```python
from build123d import *

# Parameters (mm, degrees)
F0_R      = 12.7
F1_DEPTH  = 60.325
F2_R      = 3.302
F3_W      = 57.4852150798
F3_H      = 22.3266
F4_DEPTH  = 57.151
F3_W_2    = 22.8455264698
F3_H_2    = 41.275
F3_W_3    = 20.32
F3_W_4    = 13.4658747114
F5_DEPTH  = 34.798
F6_R      = 6.35
F7_DEPTH  = 22.353
F8_R      = 5.08
F9_R      = 7.874
F11_DEPTH = 19.05


with BuildPart() as f1:
    # F0 (on Front) → F1 (new body)
    with BuildSketch(Plane.XZ):
        with BuildLine():
            Line((117.2464, 0), (22.352, 0))
            ThreePointArc((22.352, 0), (-15.8052507731, 15.8052507731), (0, -22.352))
            Line((0, -22.352), (194.2084, -22.352))
            Line((194.2084, -22.352), (194.2084, 0))
            Line((194.2084, 0), (150.0886, 0))
            Line((150.0886, 0), (150.0886, 34.798))
            Line((150.0886, 34.798), (129.7686, 34.798))
            ThreePointArc((129.7686, 34.798), (126.786603396, 16.2190014787), (117.2464, 0))
        make_face()
        Circle(F0_R, mode=Mode.SUBTRACT)
    extrude(amount=F1_DEPTH)

    # F2
    f2_edges = [f1.edges().sort_by_distance(p)[0] for p in [
        (22.352, -30.1625, 0),
        (150.0886, -30.1625, 0),
    ]]
    fillet(f2_edges, radius=F2_R)

    # F3 (on face) → F4 (cut, through all)
    with BuildSketch(Plane.XY.offset(34.798)):
        with Locations((0, -30.1625)):
            Rectangle(F3_W, F3_H)
    extrude(amount=-F4_DEPTH, mode=Mode.SUBTRACT)

    # F3 (on face) → F5 (cut, through all)
    with BuildSketch(Plane.XY.offset(34.798)):
        with Locations((118.3458367651, -20.6375)):
            Rectangle(F3_W_2, F3_H_2)
        with Locations((139.9286, -20.6375)):
            Rectangle(F3_W_3, F3_H_2)
        with Locations((156.8215373557, -20.6375)):
            Rectangle(F3_W_4, F3_H_2)
    extrude(amount=-F5_DEPTH, mode=Mode.SUBTRACT)

    # F6 (on face) → F7 (cut, through all)
    with BuildSketch(Plane.XY):
        with Locations((155.3464, -22.352)):
            Circle(F6_R)
    extrude(amount=-F7_DEPTH, mode=Mode.SUBTRACT)

    # F8
    f8_edges = [f1.edges().sort_by_distance(p)[0] for p in [
        (150.0886, -50.8, 34.798),
    ]]
    fillet(f8_edges, radius=F8_R)

    # F9
    f9_edges = [f1.edges().sort_by_distance(p)[0] for p in [
        (194.2084, -30.1625, 0),
    ]]
    fillet(f9_edges, radius=F9_R)

    # F10 (on face) → F11 (cut)
    with BuildSketch(Plane.XZ.offset(60.325)):
        Polygon((117.2464, -22.352), (117.2464, 0), (85.852, 0), (91.8464, -22.352), align=None)
    extrude(amount=-F11_DEPTH, mode=Mode.SUBTRACT)


solid = f1.part
```
Read the model definition and answer for the solid it produces. Units are mm, in the model's axes. A direction names the side the tool comes from. Give positions to 0.01 mm unless a question says otherwise; leave off trailing zeros. Write each loop counter-clockwise with the first axis right and the second up, starting at its lowest first coordinate (ties: lowest second). Pieces come first, ordered by that corner, then holes. Notation, with made-up numbers: (37.5, -33) - (46.5, -33) arc R29 cw to (46.5, 3) - close; hole circle Ø10 at (76, 85.25). An arc over 180 degrees is marked (long way). Write item = value, one per line. Start each with the question number.
Item 1: Find section C-C (z = -3.5). Give the vertices of the cut face in (x, y) (3 decimals).
Item 2: Find the intervals of material crossed by probe 1 along Y at (x, z) = (-9, 10) (3 decimals); probe 2 along Z at (x, y) = (0, -54); probe 3 along Y at (x, z) = (130.5, 15) (3 decimals), in increasing order. Write a range as [from, to].
Item 3: Find section D-D (y = -6). Give the vertices of the cut face in (x, z).
Item 4: A tool of negligible diameter and unlimited length cuts with its end or side. For faces 1 (the flat face through (9, -41.326, -10)), 2 (the flat face through (139, -41.275, 18)), 3 (the flat face through (147, -60.325, 0)), 4 (the flat face through (101, -41.275, -11)), from which of +Z, -Z, +X, -X, +Y, -Y can it reach the whole face along a straight path? Write none if from no direction.
Item 5: The mould has two halves that part along X. Classify faces 5 (the cylindrical face through (-16.31, -9.367, 15.284)), 6 (the cylindrical face through (161.4, -20.44, -11.02)), 7 (the flat face through (117.246, -51, -11)), 8 (the flat face through (96, -30, -22.352)): +X half, -X half, draft (parallel to the pull), parting line (faces both ways), or undercut.
Item 6: Each of these flat-tipped pins is pushed along its axis until it touches: P1, Ø21, axis at y = -55.5, z = 14, coming from the +X side; P2, Ø14.5, axis at x = 155.35, y = -22.35, coming from the -Z side; P3, Ø9.5, axis at y = -51.5, z = -13, coming from the -X side; P4, Ø20.5, axis at x = 0, z = 0, coming from the -Y side. Where does it stop, or does it pass through?
Item 7: Find section B-B (x = 7). Give the vertices of the cut face in (y, z) (3 decimals).
Item 8: Find section A-A (y = -56). Give the vertices of the cut face in (x, z), then the cut area to 3 significant figures.
Response:
q1.outline = (-22.076, -60.325) - (-12.208, -60.325) - (-12.208, -41.326) - (-22.076, -41.326) - close; (-22.076, -18.999) - (-12.208, -18.999) - (-12.208, 0) - (-22.076, 0) - close; (12.208, -60.325) - (86.791, -60.325) - (86.791, -41.275) - (117.246, -41.275) - (117.246, -60.325) - (192.882, -60.325) - (192.882, 0) - (12.208, 0) - (12.208, -18.999) - (28.743, -18.999) - (28.743, -41.326) - (12.208, -41.326) - close; hole circle Ø12.7 at (155.346, -22.352)
q2.probe_1 = [-60.325, -41.326], [-18.999, 0]
q2.probe_2 = [-22.35, -12.7], [12.7, 22.35]
q2.probe_3 = [-60.325, -41.275]
q3.outline = (0, -22.35) - (194.21, -22.35) - (194.21, -7.87) arc R7.87 ccw to (186.33, 0) - (25.44, 0) arc R3.3 cw to (22.17, 2.88) arc R22.35 ccw (long way) to start; hole circle Ø25.4 at (0, 0)
q4.face_1 = +Z, -Z, -X
q4.face_2 = +Z, +X, -X, +Y
q4.face_3 = +Z, -Z, +X, -X, -Y
q4.face_4 = +Z, -Y
q5.face_5 = parting line
q5.face_6 = undercut
q5.face_7 = undercut
q5.face_8 = draft
q6.P1 = 150.09
q6.P2 = -22.35
q6.P3 = -20.77
q6.P4 = through
q7.outline = (-60.325, -22.352) - (-41.326, -22.352) - (-41.326, -10.597) - (-60.325, -10.597) - close; (-60.325, 10.597) - (-41.326, 10.597) - (-41.326, 21.228) - (-60.325, 21.228) - close; (-18.999, -22.352) - (0, -22.352) - (0, -10.597) - (-18.999, -10.597) - close; (-18.999, 10.597) - (0, 10.597) - (0, 21.228) - (-18.999, 21.228) - close
q8.outline = (0, -22.35) - (91.85, -22.35) - (85.85, 0) - (25.44, 0) arc R3.3 cw to (22.17, 2.88) arc R22.35 ccw (long way) to start; (117.25, -22.35) - (194.21, -22.35) - (194.21, -7.87) arc R7.87 ccw to (186.33, 0) - (153.39, 0) arc R3.3 cw to (150.09, 3.3) - (150.09, 29.72) arc R5.08 ccw to (145.01, 34.8) - (129.77, 34.8) arc R50.8 cw to (117.25, 0) - close; hole circle Ø25.4 at (0, 0)
q8.area = 5,200 mm²
